Check sheet for the modelled part. Datum: model origin and axes. Units: mm. Face numbers are marked on the shaded views. A direction names the side the tool comes from. Round coordinates to 2 decimals unless told otherwise and drop trailing zeros. Loops run counter-clockwise (first coordinate to the right, second up) from the corner with the lowest first, then second, coordinate; pieces in that order, holes last. Notation, with made-up numbers: M 4,56 L 17,56 A12 ccw 17,65 Z; hole C 52.25,44.25 d1. An arc over 180 degrees is marked long. Write item = value, one per line. Start each with the question number.
(1) Cross-section at D-D on z = 4.15. Record the boundary of the cut face in (x, y), plus the area to 3 significant figures.
(2) Scan lines: L1, parallel to Y at x = 0, z = 5; L2, parallel to Z at x = 5, y = 0.75; L3, parallel to X at y = 1.25, z = 4.15. Record each from-to range of solid material in increasing order. Write a range as from..to.
(3) Set-up check for the marked faces 1 and 2: record each of +Z, -Z, +X, -X, +Y, -Y from which the full face is reachable in a straight line by a thin tool's end or side.
(4) Go/stop test with flat-tipped pins: P1, Ø1.5, axis at y = -5.5, z = 2, coming from the +X side; P2, Ø1.5, axis at x = 5.5, z = 0.5, coming from the -Y side; P3, Ø1, axis at y = 5, z = 4.5, coming from the -X side. Record where each tip stops, or that it passes through.
(5) Mould release check, pull along X, two halves, no side actions. Record for the marked faces 3, 4 and 5: pulls with the +X half, pulls with the -X half, needs draft (parallel to the pull), parting line crosses it, or undercut.
(6) Cross-section at A-A on y = 0. Record the boundary of the cut face in (x, z).
(7) Cross-section at C-C on z = 2.45. Record the boundary of the cut face in (x, y).
from build123d import *

# Parameters (mm, degrees)
F0_R     = 9
F1_DEPTH = 2
F2_R     = 4
F3_DEPTH = 4
F4_R     = 2.5
F5_DEPTH = 3
F6_SIZE  = 0.5


with BuildPart() as f1:
    # F0 (on Top) → F1 (new body)
    with BuildSketch(Plane.XY):
        Circle(F0_R)
    extrude(amount=F1_DEPTH)

    # F2 (on face) → F3 (join)
    with BuildSketch(Plane.XY.offset(2)):
        Circle(F2_R)
    extrude(amount=F3_DEPTH)

    # F4 (on face) → F5 (cut)
    with BuildSketch(Plane.XY.offset(6)):
        Circle(F4_R)
    extrude(amount=-F5_DEPTH, mode=Mode.SUBTRACT)

    # F6
    f6_edges = [f1.edges().sort_by_distance(p)[0] for p in [
        (-9, 0, 2),
    ]]
    chamfer(f6_edges, length=F6_SIZE)


solid = f1.part
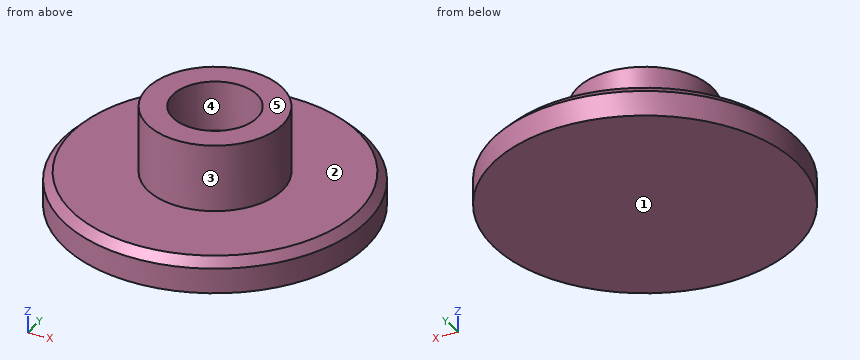
Result:
q1.outline = C 0,0 d8; hole C 0,0 d5
q1.area = 30.6 mm^2
q2.L1 = -4..-2.5, 2.5..4
q2.L2 = 0..2
q2.L3 = -3.8..-2.17, 2.17..3.8
q3.face_1 = -Z, +X, -X, +Y, -Y
q3.face_2 = +Z
q4.P1 = 7.52
q4.P2 = -7.64
q4.P3 = through
q5.face_3 = parting line crosses it
q5.face_4 = undercut
q5.face_5 = needs draft
q6.outline = M -9,0 L 9,0 L 9,1.5 L 8.5,2 L 4,2 L 4,6 L 2.5,6 L 2.5,3 L -2.5,3 L -2.5,6 L -4,6 L -4,2 L -8.5,2 L -9,1.5 Z
q7.outline = C 0,0 d8
